Could you check a few things on this model? Use its own coordinates, in mm. Face numbers are marked on the shaded views. A direction names the side the tool comes from. Round coordinates to 2 decimals unless told otherwise and drop trailing zeros. Loops run counter-clockwise (first coordinate to the right, second up) from the corner with the lowest first, then second, coordinate; pieces in that order, holes last. Notation, with made-up numbers: M 28,-6 L 71,-6 A19 ccw 71,7 Z; hole C 14.5,0 d7. An arc over 180 degrees is marked long. Answer in a Markdown table with one row per item.
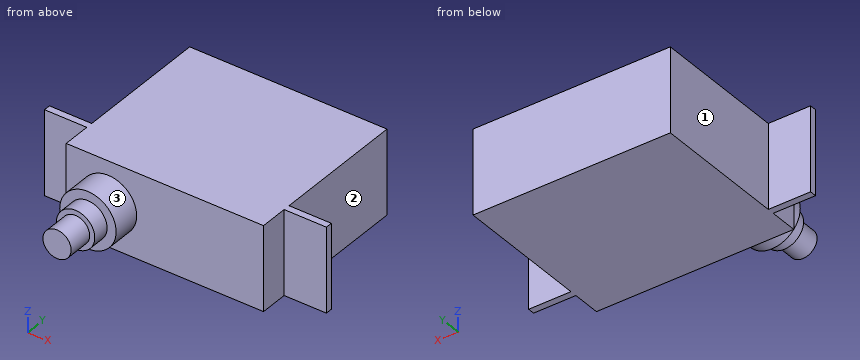
```python
from build123d import *

# Parameters (mm, degrees)
BOSS_EXTRUDE1_DEPTH = 4.7625
BOSS_EXTRUDE3_DEPTH = 3.175
SKETCH2_4_R         = 1.5875
BOSS_EXTRUDE4_DEPTH = 7.9375
SKETCH4_R           = 2.159
BOSS_EXTRUDE5_DEPTH = 1.905


with BuildPart() as part:
    # Sketch1 → Boss-Extrude1 (new, symmetric)
    with BuildSketch(Plane.XY):
        Polygon((-4.7625, 0), (0, 0), (0, 15.113), (22.225, 15.113), (22.225, 0), (26.9875, 0), (26.9875, -0.762), (22.225, -0.762), (22.225, -3.937), (7.9375, -3.937), (1.5875, -3.937), (0, -3.937), (0, -0.762), (-4.7625, -0.762), align=None)
    extrude(amount=BOSS_EXTRUDE1_DEPTH, both=True)

    # Sketch2 → Boss-Extrude3 (add)
    with BuildSketch(Plane.XZ.offset(3.937)):
        with BuildLine():
            ThreePointArc((3.175, 0), (4.7625, 1.5875), (6.35, 0))
            Line((6.35, 0), (7.9375, 0))
            ThreePointArc((7.9375, 0), (4.7625, 3.175), (1.5875, 0))
            Line((1.5875, 0), (3.175, 0))
        make_face()
        with BuildLine():
            Line((7.9375, 0), (6.35, 0))
            ThreePointArc((6.35, 0), (4.7625, -1.5875), (3.175, 0))
            Line((3.175, 0), (1.5875, 0))
            ThreePointArc((1.5875, 0), (4.7625, -3.175), (7.9375, 0))
        make_face()
    extrude(amount=BOSS_EXTRUDE3_DEPTH)

    # Sketch2_4 → Boss-Extrude4 (add)
    with BuildSketch(Plane.XZ.offset(3.937)):
        with Locations((4.7625, 0)):
            Circle(SKETCH2_4_R)
    extrude(amount=BOSS_EXTRUDE4_DEPTH)

    # Sketch4 → Boss-Extrude5 (add)
    with BuildSketch(Plane.XZ.offset(7.112)):
        with Locations(Location((4.7625, 0, 0), (0, 0, 180))):
            Circle(SKETCH4_R)
    extrude(amount=BOSS_EXTRUDE5_DEPTH)


solid = part.part
```
1) I want a section at C-C, the plane y = 11.5. Please give me the cut outline in (x, z) (1 decimal).
Computed:
| item | result |
|---|---|
| outline | M 0,-4.8 L 22.2,-4.8 L 22.2,4.8 L 0,4.8 Z |
2) I want a section at B-B, the plane x = 15. Please give me the cut outline in (y, z), plus the area to 3 significant figures.
Computed:
| item | result |
|---|---|
| outline | M -3.94,-4.76 L 15.11,-4.76 L 15.11,4.76 L -3.94,4.76 Z |
| area | 181 mm² |
3) Which directions (+Z, -Z, +X, -X, +Y, -Y) give clear straight access to the entire face, cutting with the end or side of a thin tool? Please do the marked faces 1, 2 and 3.
Computed:
| item | result |
|---|---|
| face 1 | +Z, -Z, -X, +Y |
| face 2 | +Z, -Z, +X, +Y |
| face 3 | -Y |
4) Will these pins go through, and if not, where does the flat tip stop? P1, Ø5, axis at y = -9, z = 2, coming from the +X side; P2, Ø2.5, axis at y = -2.5, z = 2.5, coming from the -X side; P3, Ø1.5, axis at y = -7.5, z = 3.5, coming from the +X side; P4, Ø3, axis at x = 17, y = -7, coming from the -Z side.
Computed:
| item | result |
|---|---|
| P1 | stops at x = 7.92 |
| P2 | stops at x = 0 |
| P3 | stops at x = 6.15 |
| P4 | passes through |
5) I need wall thicknesses on line 1 (X direction, y = -3, z = -1.75) (3 decimals); line 2 (Y direction, x = 25, z = -0.75); line 3 (Y direction, x = 13, z = 2). Which ranges of each line are inside material? Lowest first, please.
Computed:
| item | result |
|---|---|
| line 1 | x = 0 to 22.225 |
| line 2 | y = -0.76 to 0 |
| line 3 | y = -3.94 to 15.11 |
